The listing builds one solid part. Answer for the finished solid, in the listing's coordinates (mm). Give positions to 0.01 mm unless a question says otherwise; leave off trailing zeros. Write each loop counter-clockwise with the first axis right and the second up, starting at its lowest first coordinate (ties: lowest second). Pieces come first, ordered by that corner, then holes. Notation, with made-up numbers: (14, -33) - (20, -33) arc R19 cw to (20, -12) - close; hole circle Ø5 at (-10, 84). An arc over 180 degrees is marked (long way). Return JSON: item names as keys, results as strings.
from build123d import *

# Parameters (mm, degrees)
F1_DEPTH = 1.3


with BuildPart() as f1:
    # F0 (on Front) → F1 (new body)
    with BuildSketch(Plane.XZ):
        with BuildLine():
            ThreePointArc((103.3079727003, -174.0017143415), (107.9375486889, -172.4540817784), (110.1009118369, -168.0782389711))
            Line((110.1009118369, -168.0782389711), (123.3140694013, 36.0793576773))
            ThreePointArc((123.3140694013, 36.0793576773), (121.7186870706, 40.7134537603), (117.2988791147, 42.8313274396))
            Line((117.2988791147, 42.8313274396), (-86.6861012737, 53.1740147545))
            ThreePointArc((-86.6861012737, 53.1740147545), (-91.3968478399, 51.4210035289), (-93.3575316623, 46.7928396902))
            Line((-93.3575316623, 46.7928396902), (-92.6750005064, -63.4259672216))
            add(Edge.make_bspline(
                [(-92.6750005064, -63.4259672216), (-92.6146745207, -73.1677322968), (-89.962188232, -93.9434810925), (-79.4723870211, -117.0371161404), (-76.2930011516, -119.7242526752)],
                knots=[0, 0, 0, 0, 0.5251404871, 1, 1, 1, 1], degree=3))
            Line((-76.2930011516, -119.7242526752), (-25.9811858827, -162.2465266281))
            ThreePointArc((-25.9811858827, -162.2465266281), (-22.5739765007, -164.3085989306), (-18.6956488116, -165.2140227485))
            Line((-18.6956488116, -165.2140227485), (103.3079727003, -174.0017143415))
        make_face()
        with BuildLine():
            ThreePointArc((-12.0174558833, -153.6898314953), (-14.5808883162, -150.9231381327), (-11.8141949536, -148.3597056999))
            Line((-11.8141949536, -148.3597056999), (-5.3496916575, -148.6062253883))
            ThreePointArc((-5.3496916575, -148.6062253883), (-2.7862592246, -151.3729187508), (-5.5529525872, -153.9363511837))
            Line((-5.5529525872, -153.9363511837), (-12.0174558833, -153.6898314953))
        make_face(mode=Mode.SUBTRACT)
        with BuildLine():
            ThreePointArc((101.5041172504, -126.2639015913), (98.693107204, -128.7786581439), (96.1783506514, -125.9676480975))
            Line((96.1783506514, -125.9676480975), (96.5376539326, -119.5084317383))
            ThreePointArc((96.5376539326, -119.5084317383), (99.348663979, -116.9936751857), (101.8634205316, -119.8046852321))
            Line((101.8634205316, -119.8046852321), (101.5041172504, -126.2639015913))
        make_face(mode=Mode.SUBTRACT)
        with BuildLine():
            ThreePointArc((-43.0372696765, 33.8666485342), (-45.6007021093, 36.6333418967), (-42.8340087468, 39.1967743295))
            Line((-42.8340087468, 39.1967743295), (-36.3695054507, 38.9502546412))
            ThreePointArc((-36.3695054507, 38.9502546412), (-33.8060730178, 36.1835612786), (-36.5727663804, 33.6201288458))
            Line((-36.5727663804, 33.6201288458), (-43.0372696765, 33.8666485342))
        make_face(mode=Mode.SUBTRACT)
        with BuildLine():
            ThreePointArc((90.9557119012, 26.9728396088), (88.3633950976, 29.7124876865), (91.1030431753, 32.3048044901))
            Line((91.1030431753, 32.3048044901), (97.5697769586, 32.1261176179))
            ThreePointArc((97.5697769586, 32.1261176179), (100.1620937622, 29.3864695402), (97.4224456845, 26.7941527365))
            Line((97.4224456845, 26.7941527365), (90.9557119012, 26.9728396088))
        make_face(mode=Mode.SUBTRACT)
    extrude(amount=F1_DEPTH)


solid = f1.part
Item 1: A cutting plane is placed at C-C on x = -66. Determine the outline of the cut face in (y, z).
Answer below:
{"outline": "(-1.3, -128.42) - (0, -128.42) - (0, 52.13) - (-1.3, 52.13) - close"}
Item 2: A cutting plane is placed at B-B on x = 29.5. Determine the outline of the cut face in (y, z), then the cut area to 3 significant figures.
Answer below:
{"outline": "(-1.3, -168.69) - (0, -168.69) - (0, 47.28) - (-1.3, 47.28) - close", "area": "281 mm²"}
Item 3: A cutting plane is placed at A-A on y = -0.4. Give the number of separate pieces and of enclosed holes in the cut face, then the cut area to 3 significant figures.
Answer below:
{"separate pieces": "1", "enclosed holes": "4", "area": "42,900 mm²"}
Item 4: Consider L1, parallel to Z at x = -10, y = -0.75; L2, parallel to Z at x = -44, y = -0.5; L3, parallel to X at y = -1.1, z = 38. Determine where each line is inside the solid, lowest interval first.
Answer below:
{"L1": "z = -165.84 to -153.77, -148.43 to 49.29", "L2": "z = -147.02 to 34.09, 38.98 to 51.01", "L3": "x = -93.3 to -45.16, -34.43 to 123.15"}
